Job drawing, mm, ordinate dimensions from the low corner. One solid piece. A direction names the side the tool comes from. Coordinates: 2 decimals unless noted, no trailing zeros. Write each loop counter-clockwise with the first axis right and the second up, starting at its lowest first coordinate (ties: lowest second). Pieces come first, ordered by that corner, then holes. Notation, with made-up numbers: (43.25, -27) - (72.25, -27) arc R4 ccw to (72.25, -22) - close; hole circle Ø6 at (66.25, 48). An arc over 180 degrees is marked (long way). Use one line per item in the form item = value. Start each with the question number.
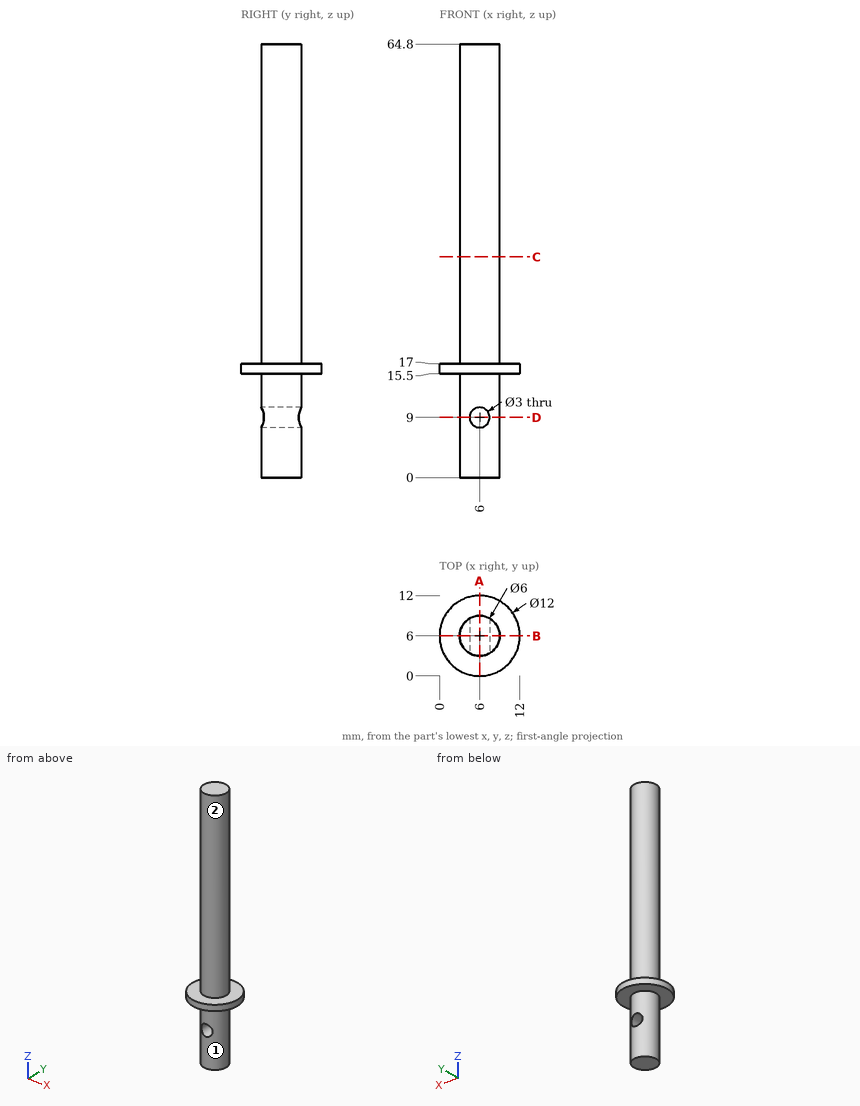
Q1. Which spindle directions (+Z, -Z, +X, -X, +Y, -Y) get a long thin tool onto all of the face, cutting with end or side? Do the marked faces 1 and 2. Say none if no direction does.
Q2. Slice it at A-A (x = 6). List the corners of the cut face in (y, z), plus the area to 3 significant figures.
Q3. Pin check, flat tips, straight feed: P1, Ø2.5, axis at x = 6, z = 9, coming from the +Y side; P2, Ø6, axis at x = 5, z = 50.5, coming from the -Y side; P3, Ø6, axis at x = 8, z = 31, coming from the +Y side; P4, Ø1.5, axis at y = 7, z = 42.5, coming from the -X side. Stop position of each tip, or through.
Q4. Slice it at D-D (z = 9). List the corners of the cut face in (x, y), plus the area to 3 significant figures.
Q5. Slice it at C-C (z = 33). List the corners of the cut face in (x, y), plus the area to 3 significant figures.
Q6. Slice it at B-B (y = 6). List the corners of the cut face in (x, z), plus the area to 3 significant figures.
Q7. Drill centre lines: probe 1 along Z at (x, y) = (6, 4); probe 2 along X at (y, z) = (6, 9); probe 3 along Z at (x, y) = (8.5, 2.75). Where is each one in solid material? Low to high.
Solution:
q1.face_1 = -Z
q1.face_2 = +Z
q2.outline = (0, 15.5) - (3, 15.5) - (3, 10.5) - (9, 10.5) - (9, 15.5) - (12, 15.5) - (12, 17) - (9, 17) - (9, 64.8) - (3, 64.8) - (3, 17) - (0, 17) - close; (3, 0) - (9, 0) - (9, 7.5) - (3, 7.5) - close
q2.area = 380 mm2
q3.P1 = through
q3.P2 = 3
q3.P3 = 9
q3.P4 = 3.01
q4.outline = (4.5, 3.4) - (4.5, 8.6) arc R3 ccw to start; (7.5, 3.4) arc R3 ccw to (7.5, 8.6) - close
q4.area = 11.1 mm2
q5.outline = circle Ø6 at (6, 6)
q5.area = 28.3 mm2
q6.outline = (0, 15.5) - (3, 15.5) - (3, 0) - (9, 0) - (9, 15.5) - (12, 15.5) - (12, 17) - (9, 17) - (9, 64.8) - (3, 64.8) - (3, 17) - (0, 17) - close; hole circle Ø3 at (6, 9)
q6.area = 391 mm2
q7.probe_1 = 0 to 7.5, 10.5 to 64.8
q7.probe_2 = 3 to 4.5, 7.5 to 9
q7.probe_3 = 15.5 to 17
